Could you check a few things on this model? Use its own coordinates, in mm. Face numbers are marked on the shaded views. Round coordinates to 2 decimals unless told otherwise and drop trailing zeros. Loops run counter-clockwise (first coordinate to the right, second up) from the corner with the lowest first, then second, coordinate; pieces in that order, holes last.
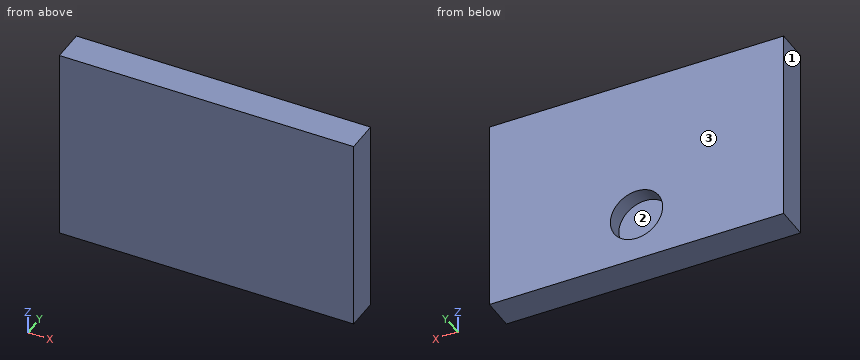
from build123d import *

# Parameters (mm, degrees)
SKETCH1_W      = 90
SKETCH1_H      = 60
EXTRUDE1_DEPTH = 10
SKETCH2_R      = 8
EXTRUDE2_DEPTH = 5


with BuildPart() as part:
    # Sketch1 → Extrude1 (new body)
    with BuildSketch(Plane(origin=(0, 0, 0), x_dir=(1, 0, 0), z_dir=(0, 1, 0))):
        with Locations((45, 30)):
            Rectangle(SKETCH1_W, SKETCH1_H)
    extrude(amount=EXTRUDE1_DEPTH)

    # Sketch2 → Extrude2 (cut)
    with BuildSketch(Plane(origin=(0, 10, 0), x_dir=(1, 0, 0), z_dir=(0, 1, 0))):
        with Locations(Location((45, 45, 0), (0, 0, 270))):
            Circle(SKETCH2_R)
    extrude(amount=-EXTRUDE2_DEPTH, mode=Mode.SUBTRACT)


solid = part.part
Item 1: If we section it at C-C, the plane x = 45: Please give me the cut outline in (y, z).
Results list:
outline: (0, -60) - (10, -60) - (10, -53) - (5, -53) - (5, -37) - (10, -37) - (10, 0) - (0, 0) - close
Item 2: If we section it at A-A, the plane z = -45: Please give me the cut outline in (x, y), then the cut area to 3 significant figures.
Results list:
outline: (0, 0) - (90, 0) - (90, 10) - (53, 10) - (53, 5) - (37, 5) - (37, 10) - (0, 10) - close
area: 820 mm2
Item 3: We'd pull the mould along X, two halves only. Please class the marked faces 1, 2 and 3: released by +X, released by -X, zero draft, split by the parting line, or undercut.
Results list:
face 1: released by -X
face 2: undercut
face 3: zero draft
Item 4: If we section it at B-B, the plane y = 9: Please give me the cut outline in (x, z).
Results list:
outline: (0, -60) - (90, -60) - (90, 0) - (0, 0) - close; hole circle Ø16 at (45, -45)
Item 5: If I drill on line 1 along X through (y, z) = (8, -45); line 2 along Y through (x, z) = (46.5, -45.5), over which ranges is the centre line in solid material (lowest first)?
Results list:
line 1: x = 0 to 37, 53 to 90
line 2: y = 0 to 5
Item 6: Will this pin go through, and if not, where does the flat tip stop? pin 1 (5 mm diameter, centred on x = 42.5, z = -42.5, fed in from +Y).
Results list:
pin 1: stops at y = 5
